Verification items for this drawing (mm, ordinates from the low corner). Round coordinates to 2 decimals unless told otherwise and drop trailing zeros. Loops run counter-clockwise (first coordinate to the right, second up) from the corner with the lowest first, then second, coordinate; pieces in that order, holes last. Notation, with made-up numbers: (85, -3) -> (109, -3) arc R19 ccw to (109, 18) -> close; hole circle Ø2 at (30.5, -29.75). An arc over 180 degrees is marked (long way). Use a Markdown table: item, result. Add a question column.
Q1. Sectioned sample at A-A, the plane z = 21. Enter the section's corners in (x, y), then the cut area to 3 significant figures.
Q2. Sectioned sample at D-D, the plane y = 0.9. Give the number of separate pieces and of enclosed holes in the cut face, then the cut area to 3 significant figures.
Q3. Gauge pin test, flat ends, axial feed: P1, Ø3.5, axis at x = 29, y = 2, coming from the +Z side; P2, Ø1.8, axis at y = 2.5, z = 2.5, coming from the -X side; P3, Ø3, axis at y = 2, z = 4, coming from the +X side. Record the tip position at first contact, or that the pin passes through.
Q4. Sectioned sample at C-C, the plane x = 19.75. Enter the section's corners in (y, z).
Q5. Material ranges on L1, parallel to X at y = 0.55, z = 62; L2, parallel to Z at x = 4.75, y = 3.6; L3, parallel to Z at x = 12.25, y = 2.9, recorded low to high.
Q6. Sectioned sample at B-B, the plane x = 24.75. Enter the section's corners in (y, z), then the cut area to 3 significant figures.
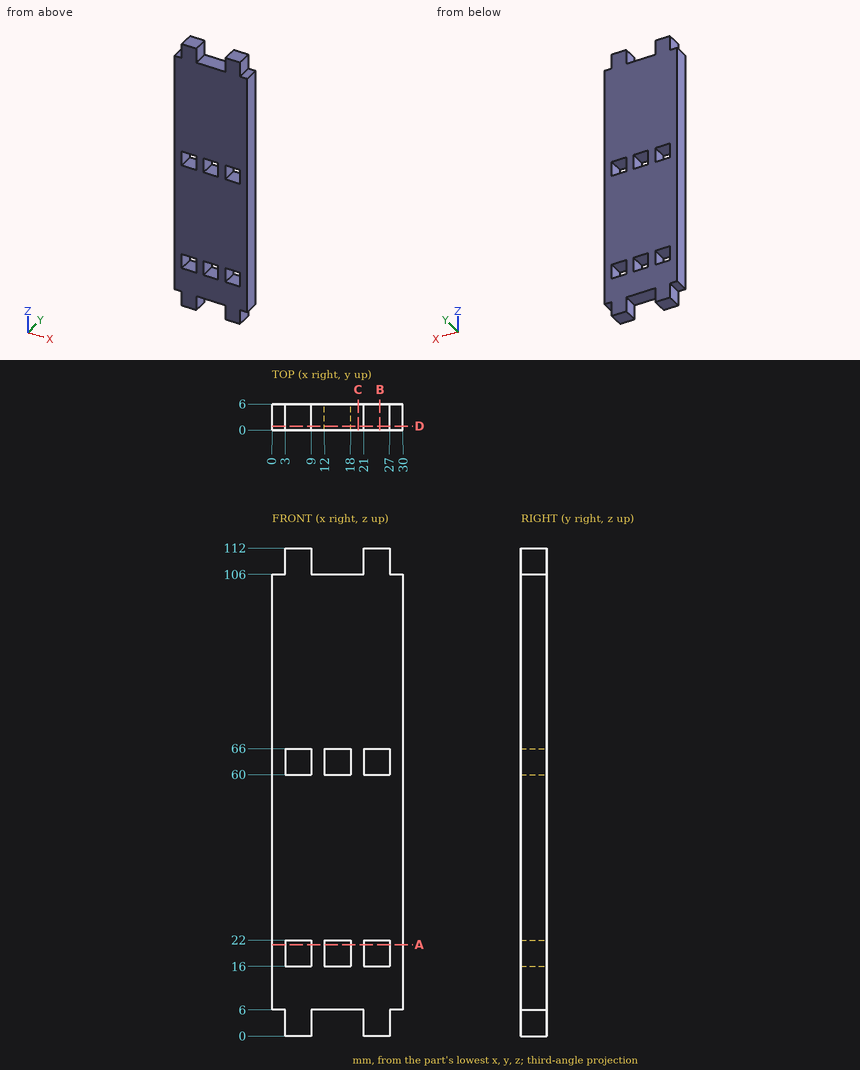
Values:
| question | item | result |
|---|---|---|
| 1 | outline | (0, 0) -> (3, 0) -> (3, 6) -> (0, 6) -> close; (9, 0) -> (12, 0) -> (12, 6) -> (9, 6) -> close; (18, 0) -> (21, 0) -> (21, 6) -> (18, 6) -> close; (27, 0) -> (30, 0) -> (30, 6) -> (27, 6) -> close |
| 1 | area | 72.0 mm^2 |
| 2 | separate pieces | 1 |
| 2 | enclosed holes | 6 |
| 2 | area | 2,930 mm^2 |
| 3 | P1 | z = 106 |
| 3 | P2 | x = 3 |
| 3 | P3 | x = 27 |
| 4 | outline | (0, 6) -> (6, 6) -> (6, 106) -> (0, 106) -> close |
| 5 | L1 | 0 to 3, 9 to 12, 18 to 21, 27 to 30 |
| 5 | L2 | 0 to 16, 22 to 60, 66 to 112 |
| 5 | L3 | 6 to 16, 22 to 60, 66 to 106 |
| 6 | outline | (0, 0) -> (6, 0) -> (6, 16) -> (0, 16) -> close; (0, 22) -> (6, 22) -> (6, 60) -> (0, 60) -> close; (0, 66) -> (6, 66) -> (6, 112) -> (0, 112) -> close |
| 6 | area | 600 mm^2 |
